Read the model definition and answer for the solid it produces. Units are mm, in the model's axes. Coordinates: 2 decimals unless noted, no trailing zeros. Write each loop counter-clockwise with the first axis right and the second up, starting at its lowest first coordinate (ties: lowest second). Pieces come first, ordered by that corner, then holes. Notation, with made-up numbers: (37, 5.25) -> (88, 5.25) arc R16 ccw to (88, 27.25) -> close; hole circle Ø6 at (27, 61.5). An arc over 180 degrees is marked (long way). Use CSV: the item, a comma, the result in double quotes.
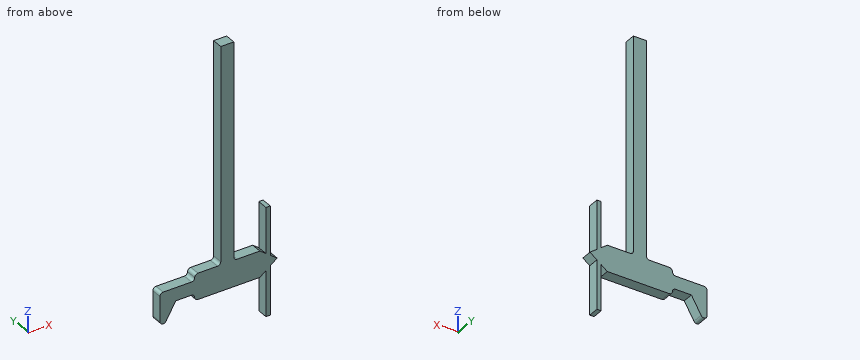
Autodesk Inventor part; units mm, degrees
ref_plane "YZ Plane" through (0, 0, 0) normal (1, 0, 0) x (0, 1, 0)
ref_plane "XZ Plane" through (0, 0, 0) normal (0, 1, 0) x (-1, 0, 0)
ref_plane "XY Plane" through (0, 0, 0) normal (0, 0, 1) x (1, 0, 0)
sketch "Náčrt1" plane through (0, 0, 0) normal (0, 1, 0) x (-1, 0, 0)
  line L0 (30, -485) -> (30, 500)
  line L1 (30, 500) -> (-30, 500)
  line L2 (-30, 500) -> (-30, -485)
  line L3 (-338.3956, 0) -> (421.6903, 0)
  line L4 (0, -1072.3) -> (0, 762.05)
  line L5 (45, -500) -> (135, -500)
  line L6 (150, -605.5) -> (150, -605.5)
  line L7 (135, -620.5) -> (-150, -620.5)
  line L8 (-150, -620.5) -> (-150, -500)
  line L9 (-178, -810.25) -> (-198, -810.25)
  line L10 (-198, -810.25) -> (-198, -310.25)
  line L11 (-198, -310.25) -> (-178, -310.25)
  line L12 (-178, -310.25) -> (-178, -810.25)
  line L13 (-150, -620.5) -> (-229.8119, -560.25)
  line L14 (-229.8119, -560.25) -> (-150, -500)
  line L15 (165, -590.5) -> (310, -590.5)
  line L16 (310, -590.5) -> (310, -545)
  line L17 (295, -530) -> (165, -530)
  line L18 (310, -590.5) -> (310, -660.0929)
  line L19 (282.0096, -667.5929) -> (237.5, -590.5)
  arc A0 (135, -620.5) -> (150, -605.5) centre (135, -605.5) ccw
  arc A1 (165, -590.5) -> (150, -605.5) centre (165, -605.5) ccw
  line L20 (150, -515) -> (150, -515)
  arc A2 (150, -515) -> (135, -500) centre (135, -515) ccw
  arc A3 (150, -515) -> (165, -530) centre (165, -515) ccw
  arc A4 (310, -545) -> (295, -530) centre (295, -545) ccw
  arc A5 (30, -485) -> (45, -500) centre (45, -485) ccw
  line L21 (-45, -500) -> (-150, -500)
  arc A6 (-45, -500) -> (-30, -485) centre (-45, -485) ccw
  line L22 (45, -500) -> (-45, -500)
  arc A7 (282.0096, -667.5929) -> (310, -660.0929) centre (295, -660.0929) ccw
  point P0 (0, 0)
  point P1 (150, -620.5)
  point P2 (150, -500)
  point P3 (310, -530)
  point P4 (150, -530)
  point P5 (-178, -521.1372)
  point P6 (-198, -536.2352)
  point P7 (-198, -584.2648)
  point P8 (-178, -599.3628)
  dimension "d0" = 60
  dimension "d2" = 300
  dimension "d3" = 120.5
  dimension "d4" = 20
  dimension "d5" = 500
  dimension "d7" = 189.75
  dimension "d9" = 100
  dimension "d11" = 100
  dimension "d12" = 178
  dimension "d13" = 160
  dimension "d14" = 30
  dimension "d15" = 30
  dimension "d16" = 30
  dimension "d17" = 15
  dimension "d18" = 15
  dimension "d19" = 15
  dimension "d20" = 15
  dimension "d21" = 15
  dimension "d22" = 1000
  dimension "d23" = 15
extrude "Vysunutí1" add sketch "Náčrt1" along normal blind 50
properties part number "Náčrt"
1. A cutting plane is placed at B-B (x = -99). Give the vertices of the cut face in (y, z), and give its area (4 significant figures).
Solutions:
outline,"(0, -620.5) -> (50, -620.5) -> (50, -500) -> (0, -500) -> close"
area,"6,025 mm^2"
2. A cutting plane is placed at A-A (y = 25). Give the vertices of the cut face in (x, z).
Solutions:
outline,"(-310, -660.09) arc R15 ccw to (-282.01, -667.59) -> (-237.5, -590.5) -> (-165, -590.5) arc R15 cw to (-150, -605.5) arc R15 ccw to (-135, -620.5) -> (150, -620.5) -> (178, -599.36) -> (178, -810.25) -> (198, -810.25) -> (198, -584.26) -> (229.81, -560.25) -> (198, -536.24) -> (198, -310.25) -> (178, -310.25) -> (178, -521.14) -> (150, -500) -> (45, -500) arc R15 cw to (30, -485) -> (30, 500) -> (-30, 500) -> (-30, -485) arc R15 cw to (-45, -500) -> (-135, -500) arc R15 ccw to (-150, -515) arc R15 cw to (-165, -530) -> (-295, -530) arc R15 ccw to (-310, -545) -> close"
3. A cutting plane is placed at C-C (z = 134). Give the vertices of the cut face in (x, y), and give its area (3 significant figures).
Solutions:
outline,"(-30, 0) -> (30, 0) -> (30, 50) -> (-30, 50) -> close"
area,"3,000 mm^2"
4. Find the intervals of material crossed by line 1 along X through (y, z) = (34.5, -483); line 2 along X through (y, z) = (18.5, 326); line 3 along Z through (x, y) = (-100.5, 37.5), in increasing order.
Solutions:
line 1,"x = -30 to 30, 178 to 198"
line 2,"x = -30 to 30"
line 3,"z = -620.5 to -500"
5. Each of these flat-tipped pins is pushed along its axis until it touches: pin 1 Ø5 at (y, z) = (5.5, 133) entering from -X; pin 2 Ø3 at (x, z) = (81.5, -556) entering from -Y; pin 3 Ø1.5 at (x, y) = (-124, 25.5) entering from +Z; pin 4 Ø10 at (y, z) = (6.5, -149) entering from +X. Where does it stop, or does it pass through?
Solutions:
pin 1,"stops at x = -30"
pin 2,"stops at y = 0"
pin 3,"stops at z = -500"
pin 4,"stops at x = 30"
